Check sheet for the drawn part. Datum: minimum x, y, z corner. Units: mm. Coordinates: 2 decimals unless noted, no trailing zeros. Loops run counter-clockwise (first coordinate to the right, second up) from the corner with the lowest first, then second, coordinate; pieces in that order, holes last.
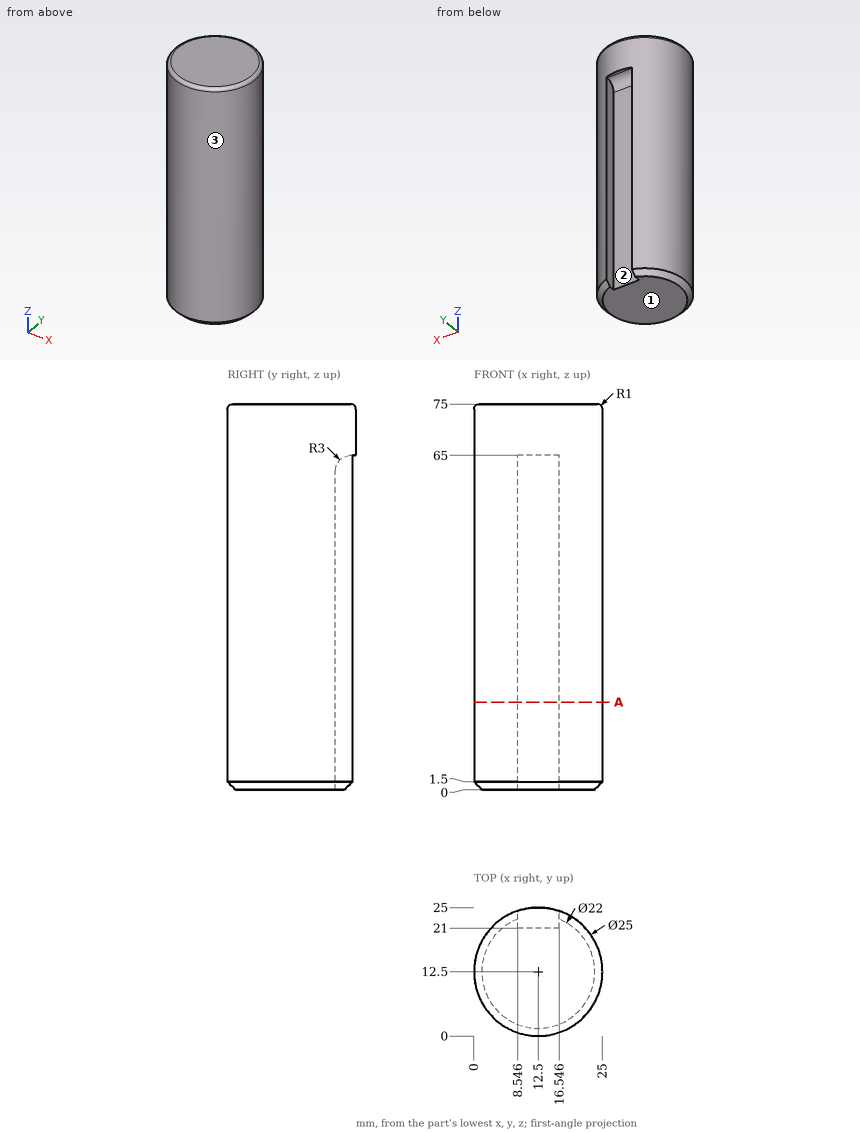
(1) Sectioned sample at A-A on z = 17. Record the cut outline in (x, y).
Findings:
outline: (8.55, 21) - (8.55, 24.36) arc R12.5 ccw (long way) to (16.55, 24.33) - (16.55, 21) - close
(2) Draft check along X on the marked faces 1, 2 and 3. Enter one of: +X half, -X half, draft (parallel to the pull), parting line (faces both ways), or undercut.
Findings:
face 1: draft
face 2: undercut
face 3: parting line
(3) Gauge pin test, flat ends, axial feed: pin 1 Ø4 at (x, z) = (13, 23) entering from +Y; pin 2 Ø2 at (x, z) = (7, 64) entering from -Y; pin 3 Ø1.5 at (x, z) = (7, 44.5) entering from -Y. Record the tip position at first contact, or that the pin passes through.
Findings:
pin 1: stops at y = 21
pin 2: stops at y = 0.84
pin 3: stops at y = 0.94
(4) Scan lines: L1, parallel to Y at x = 12, z = 28.5; L2, parallel to X at y = 22.75, z = 15 (1 decimal); L3, parallel to Y at x = 22.5, z = 59.5. Record each from-to range of solid material in increasing order.
Findings:
L1: y = 0.01 to 21
L2: x = 5.3 to 8.5, 16.5 to 19.7
L3: y = 5 to 20
